Geometry: final body of the model. Coordinates: model frame, mm. Face numbers are marked on the shaded views. A direction names the side the tool comes from. Give positions to 0.01 mm unless a question says otherwise; leave off trailing zeros. Order: outer loops, then holes, each group sorted by start corner. A loop starts at its lowest first (then second) coordinate and runs counter-clockwise, first axis right, second up. Notation, with made-up numbers: M 24.5,15 L 28.5,15 A27 ccw 28.5,47 Z; hole C 65.5,82 d4. An arc over 180 degrees is marked long. Write item = value, one per line. Start each with the question number.
from build123d import *

# Parameters (mm, degrees)
SKETCH1_W           = 40
SKETCH1_H           = 27
BOSS_EXTRUDE1_DEPTH = 30
CUT_EXTRUDE1_DEPTH  = 10
SKETCH3_R           = 2.5
CUT_EXTRUDE2_DEPTH  = 30
CUT_EXTRUDE5_START  = -10.62
CUT_EXTRUDE5_DEPTH  = 9
SKETCH10_W          = 20
SKETCH10_H          = 8.2
CUT_EXTRUDE7_DEPTH  = 6.8
SKETCH12_W          = 20
SKETCH12_H          = 8.2
CUT_EXTRUDE10_DEPTH = 6.8
FILLET1_R           = 4
SKETCH13_W          = 12.4
SKETCH13_H          = 7.4
SKETCH13_R          = 2.6
BOSS_EXTRUDE2_DEPTH = 40
CUT_EXTRUDE11_REACH = 42.436
SKETCH14_W          = 20
SKETCH14_H          = 7.4
CUT_EXTRUDE12_START = -4
SKETCH15_R          = 2.5
CUT_EXTRUDE12_DEPTH = 4
SKETCH16_R          = 2.5
CUT_EXTRUDE13_DEPTH = 4


with BuildPart() as part:
    # Sketch1 → Boss-Extrude1 (new body)
    with BuildSketch(Plane(origin=(0, 0, 0), x_dir=(1, 0, 0), z_dir=(0, 1, 0))):
        with Locations((-2.846153846, 4.313186813)):
            Rectangle(SKETCH1_W, SKETCH1_H)
    extrude(amount=BOSS_EXTRUDE1_DEPTH)

    # Sketch2 → Cut-Extrude1 (cut)
    with BuildSketch(Plane(origin=(0, 0, -17.813186813), x_dir=(-1, 0, 0), z_dir=(0, 0, -1))):
        Polygon((-8.086431081, 26), (-8.086431081, 4), (-0.206431081, 4), (-0.206431081, 7), (-2.866431081, 7), (-2.866431081, 8.008707537), (-0.253846154, 10.628707537), (5.946153846, 10.628707537), (8.558738773, 8.008707537), (8.558738773, 7), (5.898738773, 7), (5.898738773, 4), (13.778738773, 4), (13.778738773, 26), (5.898738773, 26), (5.898738773, 23), (8.558738773, 23), (8.558738773, 21.991292463), (5.938738773, 19.378707537), (-0.246431081, 19.378707537), (-2.866431081, 21.991292463), (-2.866431081, 23), (-0.206431081, 23), (-0.206431081, 26), align=None)
    extrude(amount=-CUT_EXTRUDE1_DEPTH, mode=Mode.SUBTRACT)

    # Sketch3 → Cut-Extrude2 (cut)
    with BuildSketch(Plane.XZ):
        with Locations(Location((10.423846154, 2.186813187, 0), (0, 0, 270))):
            Circle(SKETCH3_R)
        with Locations(Location((-16.116153846, 2.186813187, 0), (0, 0, 90))):
            Circle(SKETCH3_R)
    extrude(amount=-CUT_EXTRUDE2_DEPTH, mode=Mode.SUBTRACT)

    # Sketch8 → Cut-Extrude5 (cut)
    with BuildSketch(Plane.XZ.offset(CUT_EXTRUDE5_START)):
        with BuildLine():
            Line((4.453921531, 9.186813187), (17.153846154, 9.186813187))
            Line((17.153846154, 9.186813187), (17.153846154, -7.013186813))
            Line((17.153846154, -7.013186813), (10.423846154, -7.013186813))
            ThreePointArc((10.423846154, -7.013186813), (1.791349412, -0.994381557), (4.453921531, 9.186813187))
        make_face()
        with BuildLine():
            Line((-22.846153846, -7.013186813), (-16.116153846, -7.013186813))
            ThreePointArc((-16.116153846, -7.013186813), (-7.483657104, -0.994381557), (-10.146229224, 9.186813187))
            Line((-10.146229224, 9.186813187), (-22.846153846, 9.186813187))
            Line((-22.846153846, 9.186813187), (-22.846153846, -7.013186813))
        make_face()
    extrude(amount=-CUT_EXTRUDE5_DEPTH, mode=Mode.SUBTRACT)

    # Sketch10 → Cut-Extrude7 (cut)
    with BuildSketch(Plane.ZY.offset(-8.086431081)):
        with Locations((-7.813186813, 14.72)):
            Rectangle(SKETCH10_W, SKETCH10_H)
    extrude(amount=CUT_EXTRUDE7_DEPTH, mode=Mode.SUBTRACT)

    # Sketch12 → Cut-Extrude10 (cut)
    with BuildSketch(Plane(origin=(-13.778738773, 0, 0), x_dir=(0, 0, -1), z_dir=(1, 0, 0))):
        with Locations((7.813186813, 14.72)):
            Rectangle(SKETCH12_W, SKETCH12_H)
    extrude(amount=CUT_EXTRUDE10_DEPTH, mode=Mode.SUBTRACT)

    # Fillet1
    fillet1_edges = [part.edges().sort_by_distance(p)[0] for p in [
        (17.153846154, 24.81, 9.186813187),
        (-22.846153846, 24.81, 9.186813187),
        (17.153846154, 5.31, 9.186813187),
        (-22.846153846, 5.31, 9.186813187),
    ]]
    fillet(fillet1_edges, radius=FILLET1_R)

    # Sketch13 → Boss-Extrude2 (add)
    with BuildSketch(Plane(origin=(17.153846154, 0, 0), x_dir=(0, 0, -1), z_dir=(1, 0, 0))):
        with Locations((11.613186813, -3.7)):
            Rectangle(SKETCH13_W, SKETCH13_H)
        with Locations((11.613186813, -3.7)):
            Circle(SKETCH13_R, mode=Mode.SUBTRACT)
    extrude(amount=-BOSS_EXTRUDE2_DEPTH)

    # Sketch14 → Cut-Extrude11 (cut, up to next)
    with BuildSketch(Plane.XY.offset(-5.413186813), mode=Mode.PRIVATE) as cut_extrude11_sk1:
        with Locations((-2.846153846, -3.7)):
            Rectangle(SKETCH14_W, SKETCH14_H)
    cut_extrude11_tool1 = extrude(cut_extrude11_sk1.sketch, amount=-CUT_EXTRUDE11_REACH, mode=Mode.PRIVATE) & part.part
    add(cut_extrude11_tool1.solids().sort_by_distance((-2.846154, -3.7, -5.413187))[0], mode=Mode.SUBTRACT)

    # Sketch15 → Cut-Extrude12 (cut)
    # profile 1 of 2: a face of its own
    with BuildSketch(Plane(origin=(0, 30, 0), x_dir=(1, 0, 0), z_dir=(0, 1, 0)).offset(CUT_EXTRUDE12_START)):
        Polygon((12.790982258, -6.286813187), (15.158118361, -2.186813187), (12.790982258, 1.913186813), (8.05671005, 1.913186813), (5.689573946, -2.186813187), (8.05671005, -6.286813187), align=None)
        with Locations(Location((10.423846154, -2.186813187, 0), (0, 0, 90))):
            Circle(SKETCH15_R, mode=Mode.SUBTRACT)
    # profile 2 of 2: a face of its own
    with BuildSketch(Plane(origin=(0, 30, 0), x_dir=(1, 0, 0), z_dir=(0, 1, 0)).offset(CUT_EXTRUDE12_START)):
        Polygon((-13.749017742, -6.286813187), (-11.381881639, -2.186813187), (-13.749017742, 1.913186813), (-18.48328995, 1.913186813), (-20.850426054, -2.186813187), (-18.48328995, -6.286813187), align=None)
        with Locations(Location((-16.116153846, -2.186813187, 0), (0, 0, 90))):
            Circle(SKETCH15_R, mode=Mode.SUBTRACT)
    extrude(amount=CUT_EXTRUDE12_DEPTH, mode=Mode.SUBTRACT)

    # Sketch16 → Cut-Extrude13 (cut)
    # profile 1 of 2: a face of its own
    with BuildSketch(Plane.XZ):
        Polygon((-13.749017742, -1.913186813), (-11.381881639, 2.186813187), (-13.749017742, 6.286813187), (-18.48328995, 6.286813187), (-20.850426054, 2.186813187), (-18.48328995, -1.913186813), align=None)
        with Locations(Location((-16.116153846, 2.186813187, 0), (0, 0, 270))):
            Circle(SKETCH16_R, mode=Mode.SUBTRACT)
    # profile 2 of 2: a face of its own
    with BuildSketch(Plane.XZ):
        Polygon((12.790982258, -1.913186813), (15.158118361, 2.186813187), (12.790982258, 6.286813187), (8.05671005, 6.286813187), (5.689573946, 2.186813187), (8.05671005, -1.913186813), align=None)
        with Locations(Location((10.423846154, 2.186813187, 0), (0, 0, 270))):
            Circle(SKETCH16_R, mode=Mode.SUBTRACT)
    extrude(amount=-CUT_EXTRUDE13_DEPTH, mode=Mode.SUBTRACT)


solid = part.part
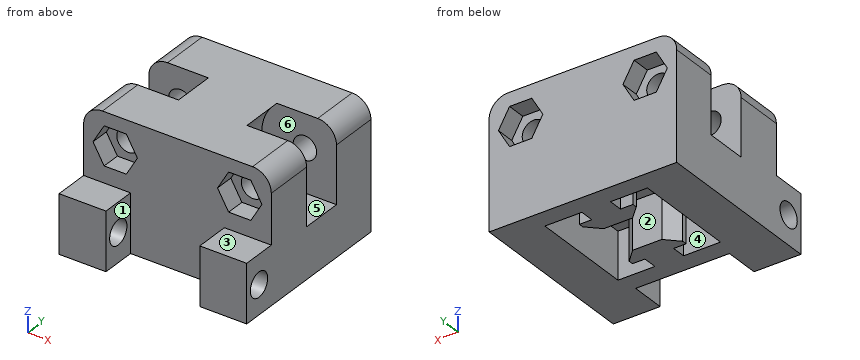
1) Cut plane C-C (z = -4). Return loops of the section in (x, y), plus the area to 3 significant figures.
2) Draft query along Z for the marked faces 4, 5 and 6. Return one class per face: pulls with the +Z half, pulls with the -Z half, needs draft (parallel to the pull), parting line crosses it, or undercut.
3) Pin query (flat end, axial travel): pin 1 Ø5 at (x, z) = (-18.5, -1.5) entering from -Y; pin 2 Ø1 at (x, z) = (8.5, 1) entering from +Y; pin 3 Ø3 at (x, z) = (8, 3) entering from -Y. Return the tip coordinate at first contact, or that it passes through.
4) Access query for the marked faces 1, 2 and 3. Directions: +Z, -Z, +X, -X, +Y, -Y. A direction counts if a zero-diameter tool reaches every point of the face in a straight line with its end or side. Return the directions, or none.
5) Cut plane D-D (y = 21). Return loops of the section in (x, z), plus the area to 3 significant figures.
6) Ray query, L1, parallel to X at y = 14, z = -7.5; L2, parallel to Y at x = 13.5, z = 7.75; L3, parallel to X at y = 18, z = -13.5. Return the intervals inside material, ascending.
7) Cut plane B-B (x = 9.5). Return loops of the section in (y, z).
8) Cut plane A-A (y = -3.7). Return loops of the section in (x, z), plus the area to 3 significant figures.
Reply:
q1.outline = M -22.85,0 L 17.15,0 L 17.15,10.62 L 1.29,10.62 L 1.29,18.82 L 3.61,18.82 L 3.61,19.62 L 17.15,19.62 L 17.15,30 L -22.85,30 L -22.85,19.62 L -9.31,19.62 L -9.31,18.82 L -6.98,18.82 L -6.98,10.62 L -22.85,10.62 Z
q1.area = 918 mm²
q2.face_4 = needs draft
q2.face_5 = pulls with the +Z half
q2.face_6 = undercut
q3.pin_1 = 0
q3.pin_2 = 26
q3.pin_3 = 4
q4.face_1 = +Z, -Z, -Y
q4.face_2 = -Z
q4.face_3 = +Z, +X, -X, -Y
q5.outline = M -22.85,-17.81 L -13.78,-17.81 L -13.78,-7.81 L -7.56,-7.81 L -7.56,-17.81 L 1.87,-17.81 L 1.87,-7.81 L 8.09,-7.81 L 8.09,-17.81 L 17.15,-17.81 L 17.15,5.19 A4 ccw 13.15,9.19 L -18.85,9.19 A4 ccw -22.85,5.19 Z; hole C -16.12,2.19 d5; hole C 10.42,2.19 d5
q5.area = 910 mm²
q6.L1 = -22.85 to -13.78, -6.98 to 1.29, 8.09 to 17.15
q6.L2 = 0 to 10.62, 19.62 to 30
q6.L3 = -22.85 to -13.78, 8.09 to 17.15
q7.outline = M -7.4,-17.81 L 30,-17.81 L 30,-1.91 L 26,-1.91 L 26,-0.14 L 19.62,-0.14 L 19.62,-6.97 L 10.62,-6.97 L 10.62,-0.14 L 4,-0.14 L 4,-1.91 L 0,-1.91 L 0,-5.41 L -7.4,-5.41 Z; M 0,6.29 L 4,6.29 L 4,4.51 L 10.62,4.51 L 10.62,9.19 L 0,9.19 Z; M 19.62,4.51 L 26,4.51 L 26,6.29 L 30,6.29 L 30,9.19 L 19.62,9.19 Z; hole C -3.7,-11.61 d5.2
q8.outline = M -22.85,-17.81 L -12.85,-17.81 L -12.85,-14.21 L -22.85,-14.21 Z; M -22.85,-9.01 L -12.85,-9.01 L -12.85,-5.41 L -22.85,-5.41 Z; M 7.15,-17.81 L 17.15,-17.81 L 17.15,-14.21 L 7.15,-14.21 Z; M 7.15,-9.01 L 17.15,-9.01 L 17.15,-5.41 L 7.15,-5.41 Z
q8.area = 144 mm²
